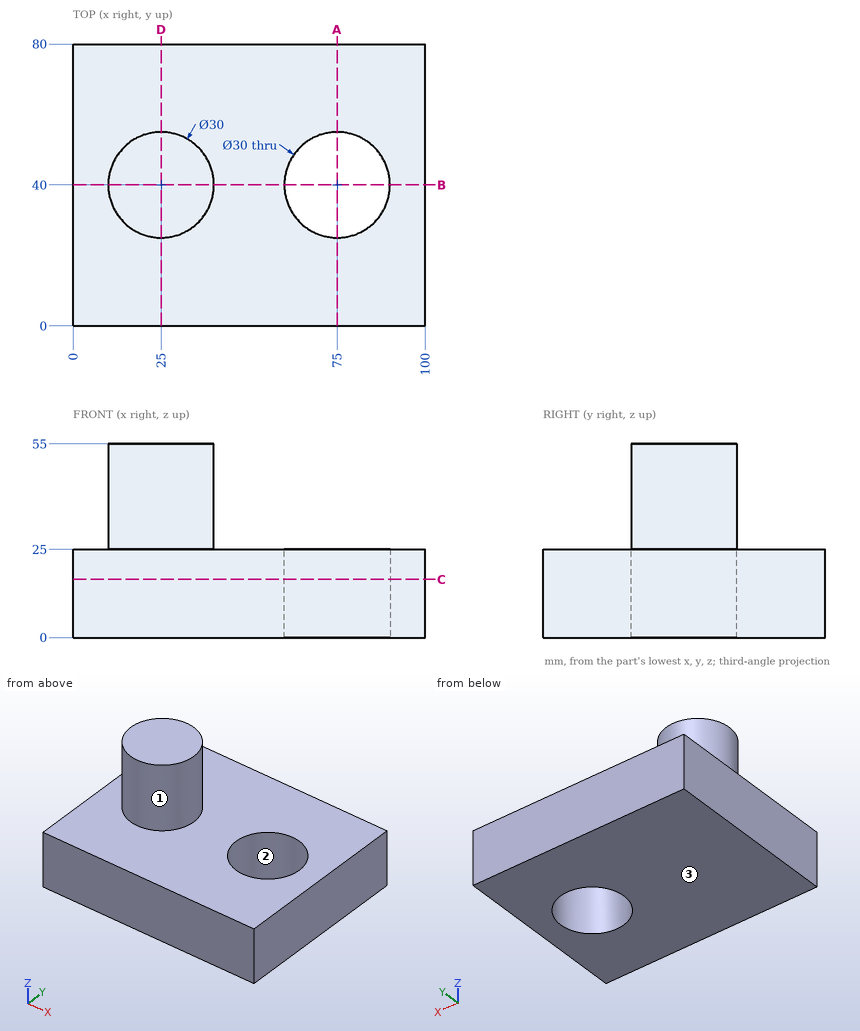
Verification items for this drawing (mm, ordinates from the low corner). Round coordinates to 2 decimals unless told otherwise and drop trailing zeros. Order: outer loops, then holes, each group sorted by start corner. A loop starts at its lowest first (then second) coordinate and runs counter-clockwise, first axis right, second up. Notation, with made-up numbers: (15.25, 32.25) - (62.25, 32.25) arc R21 ccw to (62.25, 40.25) - close; hole circle Ø3 at (-14.5, -12). An arc over 180 degrees is marked (long way). Use CSV: the item, a comma, the result in double quotes.
(1) Section check A-A on x = 75. Record the boundary of the cut face in (y, z), and give its area (3 significant figures).
Entries:
outline,"(0, 0) - (25, 0) - (25, 25) - (0, 25) - close; (55, 0) - (80, 0) - (80, 25) - (55, 25) - close"
area,"1,250 mm^2"
(2) Gauge pin test, flat ends, axial feed: pin 1 Ø2 at (x, y) = (33, 63) entering from +Z; pin 2 Ø4 at (y, z) = (61.5, 28.5) entering from +X. Record the tip position at first contact, or that the pin passes through.
Entries:
pin 1,"z = 25"
pin 2,"through"
(3) Thickness scan on probe 1 along Y at (x, z) = (75, 7.25); probe 2 along Z at (x, y) = (73, 60.5); probe 3 along X at (y, z) = (49, 14.5). Record the ranges inside material, lowest first. Write a range as from..to.
Entries:
probe 1,"0..25, 55..80"
probe 2,"0..25"
probe 3,"0..63, 87..100"
(4) Section check C-C on z = 16.5. Record the boundary of the cut face in (x, y), and give its area (3 significant figures).
Entries:
outline,"(0, 0) - (100, 0) - (100, 80) - (0, 80) - close; hole circle Ø30 at (75, 40)"
area,"7,290 mm^2"
(5) Section check B-B on y = 40. Record the boundary of the cut face in (x, z).
Entries:
outline,"(0, 0) - (60, 0) - (60, 25) - (40, 25) - (40, 55) - (10, 55) - (10, 25) - (0, 25) - close; (90, 0) - (100, 0) - (100, 25) - (90, 25) - close"
(6) Mould release check, pull along Y, two halves, no side actions. Record for the marked faces 1, 2 and 3: released by +Y, released by -Y, zero draft, split by the parting line, or undercut.
Entries:
face 1,"split by the parting line"
face 2,"undercut"
face 3,"zero draft"
(7) Section check D-D on x = 25. Record the boundary of the cut face in (y, z).
Entries:
outline,"(0, 0) - (80, 0) - (80, 25) - (55, 25) - (55, 55) - (25, 55) - (25, 25) - (0, 25) - close"
